from build123d import *

# Parameters (mm, degrees)
SKETCH1_W               = 127
SKETCH1_H               = 9.525
F_1_4_CLEARANCE_HOLE1_D = 6.7564
CUT_EXTRUDE1_REACH      = 181.858
SKETCH4_W               = 50.8
SKETCH4_H               = 2.565921067


with BuildPart() as part:
    # Sketch1 → Revolve1 (revolve)
    with BuildSketch(Plane.XY, mode=Mode.PRIVATE) as revolve1_sk:
        with Locations((63.5, 4.7625)):
            Rectangle(SKETCH1_W, SKETCH1_H)
    revolve(revolve1_sk.sketch.rotate(Axis((0, 0, 0), (0, 1, 0)), 90), axis=Axis((0, 0, 0), (0, 1, 0)))

    # 1/4 Clearance Hole1 (through all)
    with Locations(Plane(origin=(0, 9.525, 0), x_dir=(1, 0, 0), z_dir=(0, 1, 0))):
        with Locations((0, 118.745), (59.3725, 102.836186572), (102.836186572, 59.3725), (118.745, 0), (102.836186572, -59.3725), (59.3725, -102.836186572), (0, -118.745), (-59.3725, -102.836186572), (-102.836186572, -59.3725), (-118.745, 0), (-102.836186572, 59.3725), (-59.3725, 102.836186572)):
            Hole(F_1_4_CLEARANCE_HOLE1_D / 2)

    # Sketch4 → Cut-Extrude1 (cut, up to next)
    with BuildSketch(Plane(origin=(0, 9.525, 0), x_dir=(1, 0, 0), z_dir=(0, 1, 0)), mode=Mode.PRIVATE) as cut_extrude1_sk1:
        with Locations((0, -125.717039467)):
            Rectangle(SKETCH4_W, SKETCH4_H)
    cut_extrude1_tool1 = extrude(cut_extrude1_sk1.sketch, amount=-CUT_EXTRUDE1_REACH, mode=Mode.PRIVATE) & part.part
    add(cut_extrude1_tool1.solids().sort_by_distance((0, 9.525, 125.717039))[0], mode=Mode.SUBTRACT)


solid = part.part
Check sheet for the modelled part. Datum: model origin and axes. Units: mm. Round coordinates to 2 decimals unless told otherwise and drop trailing zeros. Loops run counter-clockwise (first coordinate to the right, second up) from the corner with the lowest first, then second, coordinate; pieces in that order, holes last. Notation, with made-up numbers: (56, -0.75) -> (86, -0.75) arc R24 cw to (86, 18.25) -> close; hole circle Ø5 at (-7.75, 73). An arc over 180 degrees is marked (long way). Put each result on its own line as item: value. Start each with the question number.
1. Section check A-A (z = 0). Enter the section's corners in (x, y) (3 decimals).
2. Scan lines: probe 1 along Z at (x, y) = (0, 2.5); probe 2 along Z at (x, y) = (-103.5, 6); probe 3 along X at (y, z) = (1.75, 102). Record each from-to range of solid material in increasing order.
3. Section check D-D (z = -53). Enter the section's corners in (x, y) (3 decimals), plus the area to 3 significant figures.
4. Gauge pin test, flat ends, axial feed: pin 1 (6 mm diameter, centred on x = 102.84, z = -59.37, fed in from +Y); pin 2 (8 mm diameter, centred on x = -118.745, z = 0, fed in from +Y) (3 decimals); pin 3 (1 mm diameter, centred on y = 1.5, z = 70, fed in from +X); pin 4 (1 mm diameter, centred on y = 2, z = -87.5, fed in from -X). Record the tip position at first contact, or that the pin passes through.
5. Section check B-B (y = 6). Give the number of separate pieces and of enclosed holes in the cut face, plus the area to 3 significant figures.
6. Draft check along X on faces 1 (the face through (61.86, 4.7, -105.12)), 2 (the face through (5.226, 4.829, -126.892)), 3 (the face through (-2, 0, -3)). Enter one of: +X half, -X half, draft (parallel to the pull), parting line (faces both ways), or undercut.
7. Section check C-C (x = -85). Enter the section's corners in (y, z) (3 decimals), plus the area to 3 significant figures.
Findings:
1. outline: (-127, 0) -> (-122.123, 0) -> (-122.123, 9.525) -> (-127, 9.525) -> close; (-115.367, 0) -> (115.367, 0) -> (115.367, 9.525) -> (-115.367, 9.525) -> close; (122.123, 0) -> (127, 0) -> (127, 9.525) -> (122.123, 9.525) -> close
2. probe 1: z = -127 to -122.12, -115.37 to 115.37, 122.12 to 124.43
2. probe 2: z = -73.6 to -62.68, -56.06 to 56.06, 62.68 to 73.6
2. probe 3: x = -75.66 to -62.65, -56.1 to 56.1, 62.65 to 75.66
3. outline: (-115.412, 0) -> (115.412, 0) -> (115.412, 9.525) -> (-115.412, 9.525) -> close
3. area: 2,200 mm^2
4. pin 1: passes through
4. pin 2: stops at y = 9.525
4. pin 3: stops at x = 106.3
4. pin 4: stops at x = -92.52
5. separate pieces: 1
5. enclosed holes: 12
5. area: 50,200 mm^2
6. face 1: undercut
6. face 2: parting line
6. face 3: draft
7. outline: (0, -94.361) -> (9.525, -94.361) -> (9.525, 94.361) -> (0, 94.361) -> close
7. area: 1,800 mm^2
